Can you work these out from the model? Positions are in its coordinate system, mm. Face numbers are marked on the shaded views. A direction names the side the tool comes from. Round coordinates to 2 decimals unless told otherwise and drop trailing zeros. Order: outer loops, then holes, each group sorted by start corner. A loop starts at its lowest first (then second) coordinate and runs counter-clockwise, first axis right, second up. Notation, with made-up numbers: (71.25, 71) - (99.25, 71) arc R25 cw to (99.25, 88) - close; hole circle Ø9 at (-34.5, 18.5). An arc over 180 degrees is marked (long way). Write item = value, one per line.
from build123d import *

# Parameters (mm, degrees)
BOX001_W                = 32.1
BOX001_H                = 32.1
BOX001_DEPTH            = 38.1
CYLINDER001_R           = 4
CYLINDER001_DEPTH       = 38.1
CYLINDER001_PITCH_ANGLE = 90
CYLINDER_R              = 4
CYLINDER_DEPTH          = 38.1
CYLINDER_ROLL_ANGLE     = 90
BOX_W                   = 38.1
BOX_H                   = 38.1
BOX_DEPTH               = 38.1
FILLET_R                = 1
BOX003_W                = 32.1
BOX003_H                = 32.1
BOX003_DEPTH            = 38.1
CYLINDER003_R           = 4
CYLINDER003_DEPTH       = 38.1
CYLINDER003_PITCH_ANGLE = 90
CYLINDER002_R           = 4
CYLINDER002_DEPTH       = 38.1
CYLINDER002_ROLL_ANGLE  = 90
BOX002_W                = 38.1
BOX002_H                = 38.1
BOX002_DEPTH            = 38.1
FILLET001_R             = 1


with BuildPart() as cube001:
    # Box001 → Box001 (new body)
    with BuildSketch(Plane(origin=(3, 3, 0), x_dir=(1, 0, 0), z_dir=(0, 0, 1))):
        with Locations((16.05, 16.05)):
            Rectangle(BOX001_W, BOX001_H)
    extrude(amount=BOX001_DEPTH)


with BuildPart() as cylinder001:
    # Cylinder001 → Cylinder001 (new body)
    with BuildSketch(Plane.XY):
        Circle(CYLINDER001_R)
    extrude(amount=CYLINDER001_DEPTH)


with BuildPart() as cylinder001_1:
    # Cylinder001 pitch: moved
    add(cylinder001.part.rotate(Axis((0, 0, 0), (0, 1, 0)), CYLINDER001_PITCH_ANGLE))


with BuildPart() as cylinder001_2:
    # Cylinder001 placement: moved
    add(cylinder001_1.part.moved(Location((0, 19.05, 19.05))))


with BuildPart() as cylinder:
    # Cylinder → Cylinder (new body)
    with BuildSketch(Plane.XY):
        Circle(CYLINDER_R)
    extrude(amount=CYLINDER_DEPTH)


with BuildPart() as cylinder_1:
    # Cylinder roll: moved
    add(cylinder.part.rotate(Axis((0, 0, 0), (1, 0, 0)), CYLINDER_ROLL_ANGLE))


with BuildPart() as cylinder_2:
    # Cylinder placement: moved
    add(cylinder_1.part.moved(Location((19.05, 38.1, 19.05))))


with BuildPart() as cut002:
    # Box → Box (new body)
    with BuildSketch(Plane.XY):
        with Locations((19.05, 19.05)):
            Rectangle(BOX_W, BOX_H)
    extrude(amount=BOX_DEPTH)

    # Cut: cut Cylinder
    add(cylinder_2.part, mode=Mode.SUBTRACT)

    # Cut001: cut Cylinder001
    add(cylinder001_2.part, mode=Mode.SUBTRACT)

    # Cut002: cut Cube001
    add(cube001.part, mode=Mode.SUBTRACT)


with BuildPart() as fillet_body:
    # Fillet base: copy of Cut002
    add(cut002.part)

    # Fillet
    fillet_edges = [fillet_body.edges().sort_by_distance(p)[0] for p in [
        (0, 38.1, 19.05),
        (0, 0, 19.05),
        (38.1, 38.1, 19.05),
        (38.1, 0, 19.05),
    ]]
    fillet(fillet_edges, radius=FILLET_R)


with BuildPart() as cube003:
    # Box003 → Box003 (new body)
    with BuildSketch(Plane(origin=(3, 3, 0), x_dir=(1, 0, 0), z_dir=(0, 0, 1))):
        with Locations((16.05, 16.05)):
            Rectangle(BOX003_W, BOX003_H)
    extrude(amount=BOX003_DEPTH)


with BuildPart() as cylinder003:
    # Cylinder003 → Cylinder003 (new body)
    with BuildSketch(Plane.XY):
        Circle(CYLINDER003_R)
    extrude(amount=CYLINDER003_DEPTH)


with BuildPart() as cylinder003_1:
    # Cylinder003 pitch: moved
    add(cylinder003.part.rotate(Axis((0, 0, 0), (0, 1, 0)), CYLINDER003_PITCH_ANGLE))


with BuildPart() as cylinder003_2:
    # Cylinder003 placement: moved
    add(cylinder003_1.part.moved(Location((0, 19.05, 19.05))))


with BuildPart() as cylinder002:
    # Cylinder002 → Cylinder002 (new body)
    with BuildSketch(Plane.XY):
        Circle(CYLINDER002_R)
    extrude(amount=CYLINDER002_DEPTH)


with BuildPart() as cylinder002_1:
    # Cylinder002 roll: moved
    add(cylinder002.part.rotate(Axis((0, 0, 0), (1, 0, 0)), CYLINDER002_ROLL_ANGLE))


with BuildPart() as cylinder002_2:
    # Cylinder002 placement: moved
    add(cylinder002_1.part.moved(Location((19.05, 38.1, 19.05))))


with BuildPart() as cut005:
    # Box002 → Box002 (new body)
    with BuildSketch(Plane.XY):
        with Locations((19.05, 19.05)):
            Rectangle(BOX002_W, BOX002_H)
    extrude(amount=BOX002_DEPTH)

    # Cut003: cut Cylinder002
    add(cylinder002_2.part, mode=Mode.SUBTRACT)

    # Cut004: cut Cylinder003
    add(cylinder003_2.part, mode=Mode.SUBTRACT)

    # Cut005: cut Cube003
    add(cube003.part, mode=Mode.SUBTRACT)


with BuildPart() as cut005_1:
    # Cut005 placement: moved
    add(cut005.part.moved(Location((0, 0, 38.1))))


with BuildPart() as fillet001:
    # Fillet001 base: copy of Cut005
    add(cut005_1.part)

    # Fillet001
    fillet001_edges = [fillet001.edges().sort_by_distance(p)[0] for p in [
        (0, 38.1, 57.15),
        (0, 0, 57.15),
        (38.1, 38.1, 57.15),
        (38.1, 0, 57.15),
    ]]
    fillet(fillet001_edges, radius=FILLET001_R)


with BuildPart() as fusion:
    # Fusion base: copy of Cut002
    add(cut002.part)

    # Fusion: union Fillet body, Cut005, Fillet001
    add(fillet_body.part)
    add(cut005_1.part)
    add(fillet001.part)


solid = fusion.part
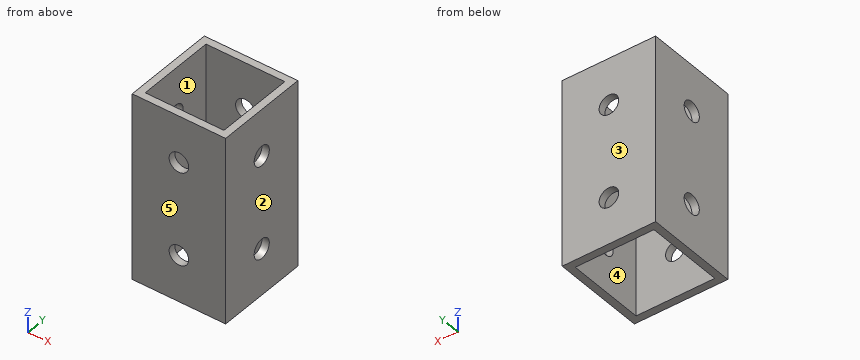
(1) On a 3-axis mill with a long thin cutter (end or side, diameter ignored), from which of +Z, -Z, +X, -X, +Y, -Y can I reach the whole of each face in a straight line? I mean the marked faces 4 and 5. Say none if no direction works.
Computed:
face_4 = +Z, -Z
face_5 = +Z, -Z, +X, -X, -Y
(2) If we section it at A-A (y = 5.5): Write out the boundary of the cut face in (x, z), plus the area to 3 significant figures.
Computed:
outline = (0, 0) - (3, 0) - (3, 76.2) - (0, 76.2) - close; (35.1, 0) - (38.1, 0) - (38.1, 76.2) - (35.1, 76.2) - close
area = 457 mm^2
(3) If we section it at D-D (x = 19.05): Write out the boundary of the cut face in (y, z), plus the area to 3 significant figures.
Computed:
outline = (0, 0) - (3, 0) - (3, 15.05) - (0, 15.05) - close; (0, 23.05) - (3, 23.05) - (3, 53.15) - (0, 53.15) - close; (0, 61.15) - (3, 61.15) - (3, 76.2) - (0, 76.2) - close; (35.1, 0) - (38.1, 0) - (38.1, 15.05) - (35.1, 15.05) - close; (35.1, 23.05) - (38.1, 23.05) - (38.1, 53.15) - (35.1, 53.15) - close; (35.1, 61.15) - (38.1, 61.15) - (38.1, 76.2) - (35.1, 76.2) - close
area = 361 mm^2
(4) Will this pin go through, and if not, where does the flat tip stop? P1, Ø13, axis at y = 19.05, z = 57.15, coming from the -X side.
Computed:
P1 = 0
(5) If I drill on line 1 (Z direction, x = 19.05, y = 37.2); line 2 (X direction, y = 5, z = 23), over which ranges is the centre line in solid material (lowest first)? Write a range as from..to.
Computed:
line_1 = 0..15.05, 23.05..53.15, 61.15..76.2
line_2 = 0..3, 35.1..38.1
(6) If we section it at B-B (z = 19.05): Write out the boundary of the cut face in (x, y).
Computed:
outline = (0, 0) - (15.05, 0) - (15.05, 3) - (3, 3) - (3, 15.05) - (0, 15.05) - close; (0, 23.05) - (3, 23.05) - (3, 35.1) - (15.05, 35.1) - (15.05, 38.1) - (0, 38.1) - close; (23.05, 0) - (38.1, 0) - (38.1, 15.05) - (35.1, 15.05) - (35.1, 3) - (23.05, 3) - close; (23.05, 35.1) - (35.1, 35.1) - (35.1, 23.05) - (38.1, 23.05) - (38.1, 38.1) - (23.05, 38.1) - close
(7) Thinking about a two-plate mould opening in Y: for the marked faces 1, 2 and 3, which applies, +Y half, -Y half, draft (parallel to the pull), parting line (faces both ways), or undercut?
Computed:
face_1 = undercut
face_2 = draft
face_3 = +Y half
